Verification items for this drawing (mm, ordinates from the low corner). Round coordinates to 2 decimals unless told otherwise and drop trailing zeros. Loops run counter-clockwise (first coordinate to the right, second up) from the corner with the lowest first, then second, coordinate; pieces in that order, holes last. Notation, with made-up numbers: (84, 85.25) - (101, 85.25) arc R18 cw to (101, 97.25) - close; hole circle Ø8 at (-8, 72). An arc over 180 degrees is marked (long way). Put each result on its own line as item: value.
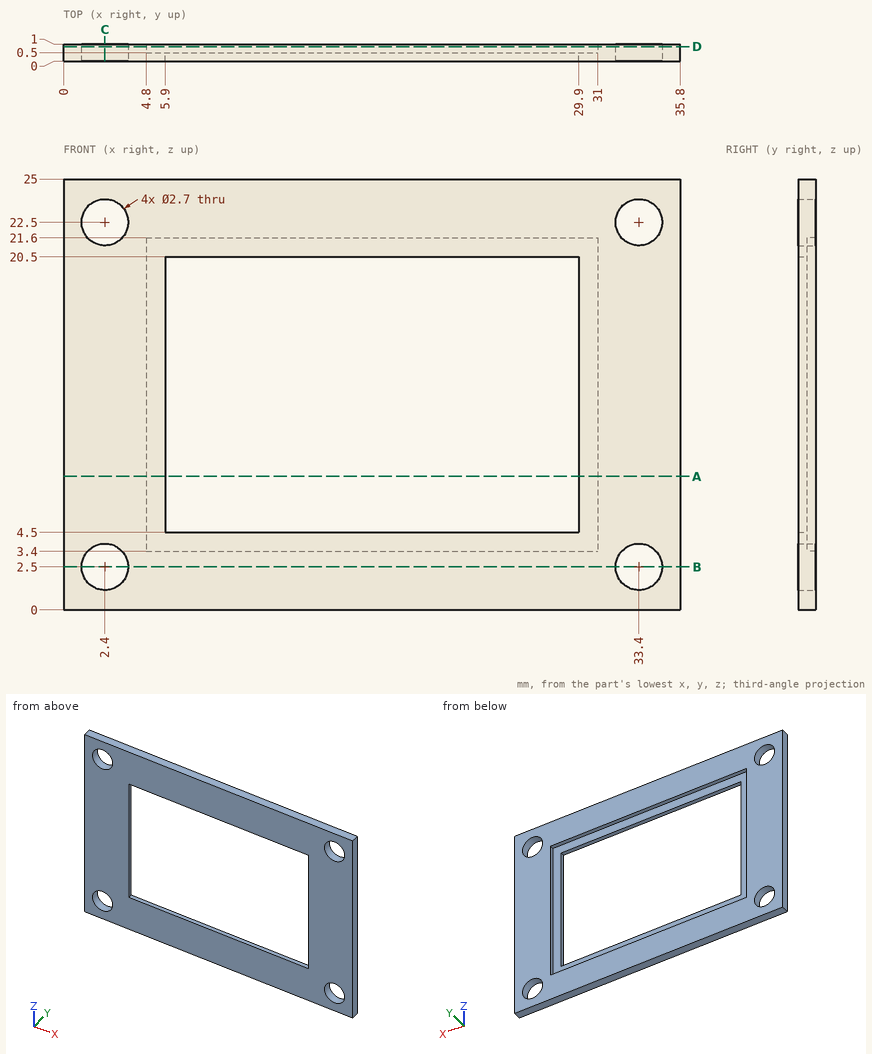
Item 1: Thickness scan on line 1 (X direction, y = 0.7, z = 2.5); line 2 (Z direction, x = 2.4, y = 0.5); line 3 (Z direction, x = 14, y = 0.2). Record the ranges inside material, lowest first. Write a range as from..to.
Filled sheet:
line 1: 0..1.05, 3.75..32.05, 34.75..35.8
line 2: 0..1.15, 3.85..21.15, 23.85..25
line 3: 0..4.5, 20.5..25
Item 2: Section check B-B on z = 2.5. Enter the section's corners in (x, y), then the cut area to 3 significant figures.
Filled sheet:
outline: (0, 0) - (1.05, 0) - (1.05, 1) - (0, 1) - close; (3.75, 0) - (32.05, 0) - (32.05, 1) - (3.75, 1) - close; (34.75, 0) - (35.8, 0) - (35.8, 1) - (34.75, 1) - close
area: 30.4 mm²
Item 3: Section check A-A on z = 7.75. Enter the section's corners in (x, y).
Filled sheet:
outline: (0, 0) - (5.9, 0) - (5.9, 0.5) - (4.8, 0.5) - (4.8, 1) - (0, 1) - close; (29.9, 0) - (35.8, 0) - (35.8, 1) - (31, 1) - (31, 0.5) - (29.9, 0.5) - close
Item 4: Go/stop test with flat-tipped pins: pin 1 (4.5 mm diameter, centred on x = 33.4, z = 2.5, fed in from +Y); pin 2 (14.5 mm diameter, centred on x = 12.5, z = 14, fed in from +Y). Record where each tip stops, or that it passes through.
Filled sheet:
pin 1: y = 1
pin 2: y = 0.5
Item 5: Section check D-D on y = 0.85. Enter the section's corners in (x, z), then the cut area to 3 significant figures.
Filled sheet:
outline: (0, 0) - (35.8, 0) - (35.8, 25) - (0, 25) - close; hole circle Ø2.7 at (2.4, 2.5); hole circle Ø2.7 at (2.4, 22.5); hole (4.8, 3.4) - (31, 3.4) - (31, 21.6) - (4.8, 21.6) - close; hole circle Ø2.7 at (33.4, 2.5); hole circle Ø2.7 at (33.4, 22.5)
area: 395 mm²
Item 6: Section check C-C on x = 2.4. Enter the section's corners in (y, z), then the cut area to 3 significant figures.
Filled sheet:
outline: (0, 0) - (1, 0) - (1, 1.15) - (0, 1.15) - close; (0, 3.85) - (1, 3.85) - (1, 21.15) - (0, 21.15) - close; (0, 23.85) - (1, 23.85) - (1, 25) - (0, 25) - close
area: 19.6 mm²
